Verification items for this drawing (mm, ordinates from the low corner). A direction names the side the tool comes from. Give positions to 0.01 mm unless a question says otherwise; leave off trailing zeros. Order: outer loops, then holes, each group sorted by start corner. A loop starts at its lowest first (then second) coordinate and runs counter-clockwise, first axis right, second up. Notation, with made-up numbers: M -16.5,-7 L 14.5,-7 A24 cw 14.5,8 Z; hole C 20,54.5 d7. An arc over 180 degrees is marked long. Answer as a JSON object with one key per item and string values.
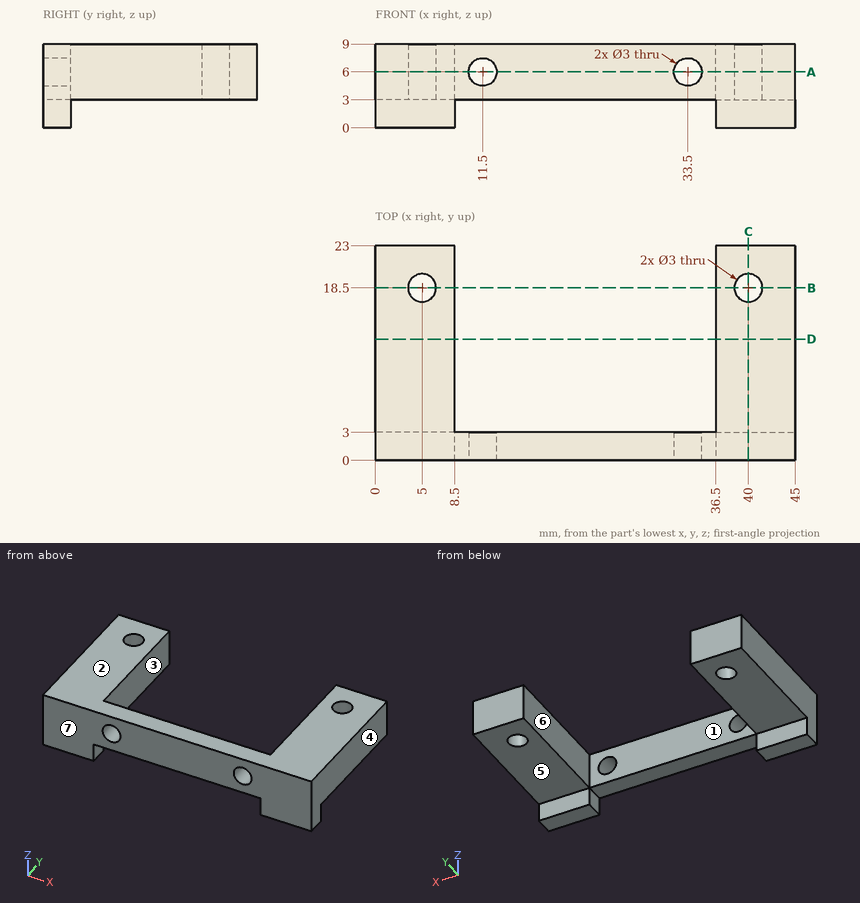
Q1. Section check D-D on y = 13. Record the cut outline in (x, z).
Resolved:
{"outline": "M 0,3 L 8.5,3 L 8.5,9 L 0,9 Z; M 36.5,3 L 45,3 L 45,9 L 36.5,9 Z"}
Q2. Tool access check on the marked faces 5, 6 and 7. Record the directions out of +Z, -Z, +X, -X, +Y, -Y that give a thin tool (end or side, any length) a straight path to the whole face; none if there is none.
Resolved:
{"face 5": "-Z, +X, -X, +Y", "face 6": "+Z, -Z, +Y", "face 7": "+Z, -Z, +X, -X, -Y"}
Q3. Section check B-B on y = 18.5. Record the cut outline in (x, z).
Resolved:
{"outline": "M 0,3 L 3.5,3 L 3.5,9 L 0,9 Z; M 6.5,3 L 8.5,3 L 8.5,9 L 6.5,9 Z; M 36.5,3 L 38.5,3 L 38.5,9 L 36.5,9 Z; M 41.5,3 L 45,3 L 45,9 L 41.5,9 Z"}
Q4. Material ranges on L1, parallel to Y at x = 40, z = 6.6; L2, parallel to X at y = 8.5, z = 8.5; L3, parallel to Z at x = 11.5, y = 1.7, recorded low to high.
Resolved:
{"L1": "y = 0 to 17, 20 to 23", "L2": "x = 0 to 8.5, 36.5 to 45", "L3": "z = 3 to 4.5, 7.5 to 9"}
Q5. Section check C-C on x = 40. Record the cut outline in (y, z), then the cut area to 3 significant figures.
Resolved:
{"outline": "M 0,0 L 3,0 L 3,3 L 17,3 L 17,9 L 0,9 Z; M 20,3 L 23,3 L 23,9 L 20,9 Z", "area": "129 mm²"}
Q6. Section check A-A on z = 6. Record the cut outline in (x, y), then the cut area to 3 significant figures.
Resolved:
{"outline": "M 0,0 L 10,0 L 10,3 L 8.5,3 L 8.5,23 L 0,23 Z; M 13,0 L 32,0 L 32,3 L 13,3 Z; M 35,0 L 45,0 L 45,23 L 36.5,23 L 36.5,3 L 35,3 Z; hole C 5,18.5 d3; hole C 40,18.5 d3", "area": "443 mm²"}
Q7. Release check for a two-part mould opening along X. For the marked faces 1, 2, 3 and 4 record: +X half, -X half, draft (parallel to the pull), parting line (faces both ways), or undercut.
Resolved:
{"face 1": "undercut", "face 2": "draft", "face 3": "undercut", "face 4": "+X half"}
Q8. Gauge pin test, flat ends, axial feed: pin 1 Ø5 at (x, z) = (17.5, 6) entering from +Y; pin 2 Ø0.9 at (x, y) = (26, 1) entering from -Z. Record the tip position at first contact, or that the pin passes through.
Resolved:
{"pin 1": "stops at y = 3", "pin 2": "stops at z = 3"}
